Here's how the part is built. I have some questions about the finished solid (model axes, mm). A direction names the side the tool comes from. Round coordinates to 2 decimals unless told otherwise and drop trailing zeros. Write each loop counter-clockwise with the first axis right and the second up, starting at its lowest first coordinate (ties: lowest second). Pieces come first, ordered by that corner, then holes. Notation, with made-up numbers: M -20.75,65.25 L -5.75,65.25 A29 ccw -5.75,85.25 Z; hole C -34,19 d1. An arc over 180 degrees is marked long. Use one line per item in the form item = value. Start each with the question number.
Q1. I need wall thicknesses on line 1 along Y through (x, z) = (0, 3.95); line 2 along Y through (x, z) = (0, 0.1); line 3 along Y through (x, z) = (0, 2.75). Which ranges of each line are inside material? Lowest first, please. Write a range as from..to.
Q2. I'm going to push a flat-ended pin straight in: pin 1 Ø6.5 at (x, y) = (0, 0) entering from +Z. Where does the tip first touch, or does it pass through?
Q3. I want a section at C-C on z = 0.55. List the corners of the cut face in (x, y) for me, and give its area (3 significant figures).
Q4. I want a section at D-D on y = -2.75. List the corners of the cut face in (x, z) for me, and give its area (3 significant figures).
Q5. For faces 4 (the face through (1, -3, 3.8)), 5 (the face through (-2, 2, 4)), which set-ups out of +Z, -Z, +X, -X, +Y, -Y let a thin tool reach every point of the face, with its end or its side?
Q6. I want a section at A-A on x = 0. List the corners of the cut face in (y, z) for me, and give its area (3 significant figures).
Q7. We'd pull the mould along X, two halves only. Please class faces 1 (the face through (2, 2, 0)), 2 (the face through (-1.08, -4.88, 2.38)), 3 (the face through (-3.3, -1.1, 0.2)): +X half, -X half, draft (parallel to the pull), parting line (faces both ways), or undercut.
```python
from build123d import *

# Parameters (mm, degrees)
SKETCH_1_R          = 5
EXTRUDE_1_DEPTH     = 4
SKETCH_2_R          = 5.8
EXTRUDE_2_DEPTH     = 0.8
SKETCH_3_R          = 2.5
CUT_EXTRUDE_1_DEPTH = 5
SKETCH_4_R          = 5.1
SKETCH_4_R_2        = 3.3
CUT_EXTRUDE_3_DEPTH = 0.2
SKETCH_5_R          = 4.5
SKETCH_5_R_2        = 3
CUT_EXTRUDE_4_DEPTH = 0.2


with BuildPart() as part:
    # 草圖1 → 填料-伸長1 (new body)
    with BuildSketch(Plane.XY):
        Circle(SKETCH_1_R)
    extrude(amount=EXTRUDE_1_DEPTH)

    # 草圖2 → 填料-伸長2 (add)
    with BuildSketch(Plane(origin=(0, 0, 0), x_dir=(-1, 0, 0), z_dir=(0, 0, -1))):
        Circle(SKETCH_2_R)
    extrude(amount=-EXTRUDE_2_DEPTH)

    # 草圖3 → 除料-伸長1 (cut, through all)
    with BuildSketch(Plane(origin=(0, 0, 0), x_dir=(-1, 0, 0), z_dir=(0, 0, -1))):
        Circle(SKETCH_3_R)
    extrude(amount=-CUT_EXTRUDE_1_DEPTH, mode=Mode.SUBTRACT)

    # 草圖4 → 除料-伸長3 (cut)
    with BuildSketch(Plane(origin=(0, 0, 0), x_dir=(-1, 0, 0), z_dir=(0, 0, -1))):
        Circle(SKETCH_4_R)
        Circle(SKETCH_4_R_2, mode=Mode.SUBTRACT)
    extrude(amount=-CUT_EXTRUDE_3_DEPTH, mode=Mode.SUBTRACT)

    # 草圖5 → 除料-伸長4 (cut)
    with BuildSketch(Plane.XY.offset(4)):
        Circle(SKETCH_5_R)
        Circle(SKETCH_5_R_2, mode=Mode.SUBTRACT)
    extrude(amount=-CUT_EXTRUDE_4_DEPTH, mode=Mode.SUBTRACT)


solid = part.part
```
Reported:
q1.line_1 = -5..-4.5, -3..-2.5, 2.5..3, 4.5..5
q1.line_2 = -5.8..-5.1, -3.3..-2.5, 2.5..3.3, 5.1..5.8
q1.line_3 = -5..-2.5, 2.5..5
q2.pin_1 = 4
q3.outline = C 0,0 d11.6; hole C 0,0 d5
q3.area = 86.0 mm^2
q4.outline = M -5.11,0 L -4.3,0 L -4.3,0.2 L -1.82,0.2 L -1.82,0 L 1.82,0 L 1.82,0.2 L 4.3,0.2 L 4.3,0 L 5.11,0 L 5.11,0.8 L 4.18,0.8 L 4.18,4 L 3.56,4 L 3.56,3.8 L 1.2,3.8 L 1.2,4 L -1.2,4 L -1.2,3.8 L -3.56,3.8 L -3.56,4 L -4.18,4 L -4.18,0.8 L -5.11,0.8 Z
q4.area = 33.0 mm^2
q5.face_4 = +Z
q5.face_5 = +Z, +X, -X, +Y, -Y
q6.outline = M -5.8,0 L -5.1,0 L -5.1,0.2 L -3.3,0.2 L -3.3,0 L -2.5,0 L -2.5,4 L -3,4 L -3,3.8 L -4.5,3.8 L -4.5,4 L -5,4 L -5,0.8 L -5.8,0.8 Z; M 2.5,0 L 3.3,0 L 3.3,0.2 L 5.1,0.2 L 5.1,0 L 5.8,0 L 5.8,0.8 L 5,0.8 L 5,4 L 4.5,4 L 4.5,3.8 L 3,3.8 L 3,4 L 2.5,4 Z
q6.area = 20.0 mm^2
q7.face_1 = draft
q7.face_2 = parting line
q7.face_3 = undercut
